```python
from build123d import *

# Parameters (mm, degrees)
SKETCH_1_R          = 1.600000000000001
SKETCH_1_R_2        = 1.6000000000000019
SKETCH_1_R_3        = 1.5999999999999985
EXTRUDE_1_DEPTH     = 3
EXTRUDE_2_DEPTH     = 30
CUT_EXTRUDE_1_DEPTH = 40
SKETCH_4_R          = 1.6499999999999986
SKETCH_4_R_2        = 1.6499999999999997
EXTRUDE_3_DEPTH     = 4
CUT_EXTRUDE_START   = -3
CUT_EXTRUDE_5_DEPTH = 3
EXTRUDE_4_DEPTH     = 3
FILLET_2_R          = 3
EXTRUDE_5_DEPTH     = 4
SKETCH_10_R         = 2.9999999999999996
CUT_EXTRUDE_6_DEPTH = 4
SKETCH_11_R         = 1.6500000000000008
CUT_EXTRUDE_7_DEPTH = 62.45571715470519


with BuildPart() as part:
    # 草图1 → 凸台-拉伸1 (new body)
    with BuildSketch(Plane.XY):
        with BuildLine():
            Line((-8.023322075989554, -14.631711796201198), (27.976677924010442, -14.631711796201193))
            Line((27.976677924010442, -14.631711796201193), (27.976677924010446, -38.631711796201195))
            Line((27.976677924010446, -38.631711796201195), (-8.023322075989551, -38.6317117962012))
            ThreePointArc((-8.023322075989551, -38.6317117962012), (-43.46930578748299, -14.57230150362017), (-57.14129859782335, 26.027570386525145))
            Line((-57.14129859782335, 26.027570386525145), (-34.48878313976992, 26.027570386525145))
            ThreePointArc((-34.48878313976992, 26.027570386525145), (-27.28963076602897, 1.7706236653637966), (-8.023322075989554, -14.631711796201198))
        make_face()
        with Locations((3.976677924010446, -26.6317117962012)):
            Circle(SKETCH_1_R, mode=Mode.SUBTRACT)
        with Locations(Location((15.976677924010446, -26.6317117962012, 0), (0, 0, 180))):
            Circle(SKETCH_1_R_2, mode=Mode.SUBTRACT)
        with Locations((-42.682604258715905, 20.02757038652514)):
            Circle(SKETCH_1_R_3, mode=Mode.SUBTRACT)
    extrude(amount=EXTRUDE_1_DEPTH)

    # 草图2 → 凸台-拉伸2 (add)
    with BuildSketch(Plane.XY.offset(3)):
        with BuildLine():
            Line((-20.49424577864387, -33.77498458475056), (-10.210218965484446, -13.591445522347069))
            ThreePointArc((-10.210218965484446, -13.591445522347069), (-5.231405442065514, -15.756295254952452), (-0.02587442417285965, -17.298243790895924))
            Line((-0.02587442417285965, -17.298243790895924), (-5.121581660002594, -39.370176745308015))
            ThreePointArc((-5.121581660002594, -39.370176745308015), (-12.979022025715798, -37.042696873124), (-20.49424577864387, -33.77498458475056))
        make_face()
    extrude(amount=EXTRUDE_2_DEPTH)

    # 草图3 → 切除-拉伸1 (cut)
    with BuildSketch(Plane.XY.offset(3)):
        with BuildLine():
            Line((-14.348702760927614, -28.820181203971632), (-7.456511566861831, -13.279984919997544))
            ThreePointArc((-7.456511566861831, -13.279984919997544), (-4.701142282615541, -14.38977235123981), (-1.875728376120071, -15.30668253882269))
            Line((-1.875728376120071, -15.30668253882269), (-6.561563425008877, -31.648131369774166))
            ThreePointArc((-6.561563425008877, -31.648131369774166), (-10.504001434072327, -30.368721805705025), (-14.348702760927614, -28.820181203971632))
        make_face()
    extrude(amount=CUT_EXTRUDE_1_DEPTH, mode=Mode.SUBTRACT)

    # 草图4 → 凸台-拉伸3 (add)
    with BuildSketch(Plane.XY.offset(33)):
        Polygon((-27.87837659400939, -26.811760111104594), (5.010865133497435, -38.782465127502874), (27.24217444966564, 22.297555223581274), (16.435709310627683, 26.230786871826414), (-0.6652978556555434, -20.753844167469087), (-11.941609305086462, -16.649602447561108), (-15.43021476700824, -26.234467179577372), (-26.236679906046202, -22.30123553133223), align=None)
        with Locations((20.36376431871485, 19.48020290794287)):
            Circle(SKETCH_4_R, mode=Mode.SUBTRACT)
        with Locations((0.4581919771611356, -35.20990762179707)):
            Circle(SKETCH_4_R_2, mode=Mode.SUBTRACT)
        with Locations(Location((-22.094430921700695, -27.001424181981108, 0), (0, 0, 180))):
            Circle(SKETCH_4_R, mode=Mode.SUBTRACT)
    extrude(amount=EXTRUDE_3_DEPTH)

    # 草图7 → 切除-拉伸5 (cut)
    with BuildSketch(Plane.XY.offset(3).offset(CUT_EXTRUDE_START)):
        with BuildLine():
            Line((-12.256052607879635, -12.480648485696536), (-23.582310336906296, -32.09830233199053))
            ThreePointArc((-23.582310336906296, -32.09830233199053), (-48.149194794505114, -7.53141787439181), (-57.14129859782335, 26.027570386525152))
            Line((-57.14129859782335, 26.027570386525152), (-34.48878313976992, 26.027570386525145))
            ThreePointArc((-34.48878313976992, 26.027570386525145), (-28.53154094821116, 3.794839854634926), (-12.256052607879635, -12.480648485696536))
        make_face()
    extrude(amount=CUT_EXTRUDE_5_DEPTH, mode=Mode.SUBTRACT)

    # 草图8 → 凸台-拉伸4 (add)
    with BuildSketch(Plane(origin=(0, 0, 0), x_dir=(-1, 0, 0), z_dir=(0, 0, -1))):
        with BuildLine():
            Line((-27.976677924010446, -38.631711796201195), (8.023322075989551, -38.6317117962012))
            ThreePointArc((8.023322075989551, -38.6317117962012), (-9.97667792401045, -41.090406135308655), (-27.976677924010446, -38.631711796201195))
        make_face()
    extrude(amount=-EXTRUDE_4_DEPTH)

    # 圆角2
    fillet_2_edges = [part.edges().sort_by_distance(p)[0] for p in [
        (-26.236679906046202, -22.30123553133223, 35),
    ]]
    fillet(fillet_2_edges, radius=FILLET_2_R)
    fillet_2_2_edges = [part.edges().sort_by_distance(p)[0] for p in [
        (27.24217444966564, 22.297555223581274, 35),
    ]]
    fillet(fillet_2_2_edges, radius=FILLET_2_R)
    fillet_2_3_edges = [part.edges().sort_by_distance(p)[0] for p in [
        (16.435709310627683, 26.230786871826414, 35),
    ]]
    fillet(fillet_2_3_edges, radius=FILLET_2_R)
    fillet_2_4_edges = [part.edges().sort_by_distance(p)[0] for p in [
        (27.976677924010446, -38.631711796201195, 1.5),
    ]]
    fillet(fillet_2_4_edges, radius=FILLET_2_R)
    fillet_2_5_edges = [part.edges().sort_by_distance(p)[0] for p in [
        (-23.5823103369063, -32.09830233199054, 1.5),
    ]]
    fillet(fillet_2_5_edges, radius=FILLET_2_R)
    fillet_2_6_edges = [part.edges().sort_by_distance(p)[0] for p in [
        (-12.256052607879633, -12.480648485696538, 1.5),
    ]]
    fillet(fillet_2_6_edges, radius=FILLET_2_R)
    fillet_2_7_edges = [part.edges().sort_by_distance(p)[0] for p in [
        (27.976677924010442, -14.631711796201193, 1.5),
    ]]
    fillet(fillet_2_7_edges, radius=FILLET_2_R)
    # the kernel refuses this fillet: 3 mm, written as the material it adds along each edge
    with BuildSketch(Plane(origin=(-0.6652978556555434, -20.753844167469087, 33), x_dir=(-0.93969262078591, 0.34202014332566444, 0), z_dir=(0, 0, 1))) as fillet_2_8_piece_1:
        with BuildLine():
            CenterArc((FILLET_2_R, -FILLET_2_R), FILLET_2_R, 89.99999999999999, 90.00000000000001)
            Line((5e-17, -FILLET_2_R), (-FILLET_2_R * 0.02, -FILLET_2_R))
            Line((-FILLET_2_R * 0.02, -FILLET_2_R), (-FILLET_2_R * 0.02, FILLET_2_R * 0.02))
            Line((-FILLET_2_R * 0.02, FILLET_2_R * 0.02), (FILLET_2_R, FILLET_2_R * 0.02))
            Line((FILLET_2_R, FILLET_2_R * 0.02), (FILLET_2_R, -5e-17))
        make_face()
    extrude(amount=4)
    # the kernel refuses this fillet: 3 mm, written as the material it takes off along each edge
    with BuildSketch(Plane(origin=(-11.941609305086462, -16.649602447561108, 33), x_dir=(0.9396926207859099, -0.3420201433256647, 0), z_dir=(0, 0, 1))) as fillet_2_9_piece_1:
        with BuildLine():
            CenterArc((FILLET_2_R, -FILLET_2_R), FILLET_2_R, 89.99999999999997, 90)
            Line((-2.84e-15, -FILLET_2_R), (-FILLET_2_R * 0.02, -FILLET_2_R))
            Line((-FILLET_2_R * 0.02, -FILLET_2_R), (-FILLET_2_R * 0.02, FILLET_2_R * 0.02))
            Line((-FILLET_2_R * 0.02, FILLET_2_R * 0.02), (FILLET_2_R, FILLET_2_R * 0.02))
            Line((FILLET_2_R, FILLET_2_R * 0.02), (FILLET_2_R, -5e-17))
        make_face()
    extrude(amount=11.5, mode=Mode.SUBTRACT)
    # the kernel refuses this fillet: 3 mm, written as the material it adds along each edge
    with BuildSketch(Plane(origin=(-15.43021476700824, -26.234467179577372, 33), x_dir=(0.34202014332566544, 0.9396926207859095, 0), z_dir=(0, 0, 1))) as fillet_2_10_piece_1:
        with BuildLine():
            CenterArc((FILLET_2_R, FILLET_2_R), FILLET_2_R, 180.00000000000006, 90)
            Line((-5.63e-15, FILLET_2_R), (-FILLET_2_R * 0.02, FILLET_2_R))
            Line((-FILLET_2_R * 0.02, FILLET_2_R), (-FILLET_2_R * 0.02, -FILLET_2_R * 0.02))
            Line((-FILLET_2_R * 0.02, -FILLET_2_R * 0.02), (FILLET_2_R, -FILLET_2_R * 0.02))
            Line((FILLET_2_R, -FILLET_2_R * 0.02), (FILLET_2_R, 9e-17))
        make_face()
    extrude(amount=4)

    # 草图9 → 凸台-拉伸5 (add)
    with BuildSketch(Plane.XY.offset(37.00000000000001)):
        with BuildLine():
            Line((-27.87837659400939, -26.811760111104594), (-29.094175630850113, -30.152140511419198))
            ThreePointArc((-29.094175630850113, -30.152140511419198), (-13.427826993623084, -38.27577838818826), (3.79506609665671, -42.12284552781748))
            Line((3.79506609665671, -42.12284552781748), (5.010865133497435, -38.782465127502874))
            Line((5.010865133497435, -38.782465127502874), (-27.87837659400939, -26.811760111104594))
        make_face()
    extrude(amount=-EXTRUDE_5_DEPTH)

    # 草图10 → 切除-拉伸6 (cut)
    with BuildSketch(Plane.XY.offset(37.00000000000001)):
        with Locations((3.976677924010446, -26.6317117962012)):
            Circle(SKETCH_10_R)
    extrude(amount=-CUT_EXTRUDE_6_DEPTH, mode=Mode.SUBTRACT)

    # 草图11 → 切除-拉伸7 (cut, through all)
    with BuildSketch(Plane.XY.offset(3)):
        with Locations((0.4581919771611356, -35.20990762179707)):
            Circle(SKETCH_11_R)
    extrude(amount=-CUT_EXTRUDE_7_DEPTH, mode=Mode.SUBTRACT)


solid = part.part
```
Read the model definition and answer for the solid it produces. Units are mm, in the model's axes. A direction names the side the tool comes from. Coordinates: 2 decimals unless noted, no trailing zeros. Loops run counter-clockwise (first coordinate to the right, second up) from the corner with the lowest first, then second, coordinate; pieces in that order, holes last.
(1) The part is cut by section D-D (y = 15). Determine the outline of the cut face in (x, z).
Solution:
outline: (12.35, 33) - (24.59, 33) - (24.59, 37) - (12.35, 37) - close
(2) Flat-ended cylindrical pins translate along their axes: pin 1 Ø6 at (x, y) = (18, -33) entering from +Z; pin 2 Ø8 at (y, z) = (8, 30) entering from -X; pin 3 Ø3 at (y, z) = (-17, 11) entering from -X. Find the tip coordinate at first contact, or state that the pin passes through.
Solution:
pin 1: stops at z = 3
pin 2: stops at x = 8.84
pin 3: stops at x = -12.71
(3) The mould has two halves that part along Y. Classify faces 5 (the face through (-2, -18, 33)), 6 (the face through (-10.45, -30.39, 17.79)), 7 (the face through (27.075, -15.487, 1.521)), 8 (the face through (1.22, -36.674, 34.972)): released by +Y, released by -Y, zero draft, split by the parting line, or undercut.
Solution:
face 5: zero draft
face 6: undercut
face 7: released by +Y
face 8: undercut
(4) The part is cut by section A-A (z = 16.5). Determine the outline of the cut face in (x, y).
Solution:
outline: (-20.49, -33.77) arc R67.12 ccw to (-5.12, -39.37) - (-0.03, -17.3) arc R44.47 cw to (-2.28, -16.72) - (-6.56, -31.65) arc R60 cw to (-14.35, -28.82) - (-8.05, -14.62) arc R44.47 cw to (-9.78, -13.81) arc R3 ccw to (-10.23, -13.63) - close
(5) The part is cut by section C-C (y = -21.5). Determine the outline of the cut face in (x, z).
Solution:
outline: (-17.46, 0) - (27.98, 0) - (27.98, 3) - (-1, 3) - (-1, 33) - (11.3, 33) - (11.3, 37) - (-13.71, 37) - (-13.71, 33) - (-14.24, 33) - (-14.24, 3) - (-17.46, 3) - close; hole (-11.1, 3) - (-3.65, 3) - (-3.65, 33) - (-11.1, 33) - close
(6) Consider line 1 along Z through (x, y) = (-12, -28); line 2 along X through (y, z) = (-21.5, 5.5); line 3 along Z through (x, y) = (10.5, -38). Determine where each line is inside the solid, lowest interval first.
Solution:
line 1: z = 0 to 3, 33 to 37
line 2: x = -14.24 to -11.1, -3.65 to -1
line 3: z = 0 to 3
(7) A tool of negligible diameter and unlimited length cuts with its end or side. For faces 1 (the face through (-15.43, -23.84, 17.79)), 2 (the face through (-15.985, -25.122, 34.972)), 3 (the face through (-11.244, -21.819, 17.79)), 4 (the face through (3.33, -29.56, 35.03)), from which of +Z, -Z, +X, -X, +Y, -Y can it reach the whole face along a straight path? Write none if from no direction.
Solution:
face 1: -X, +Y
face 2: +Z, +Y
face 3: none
face 4: +Z
(8) The part is cut by section B-B (x = -11). Determine the outline of the cut face in (y, z), and give its area (3 significant figures).
Solution:
outline: (-39.11, 33) - (-37.73, 33) - (-37.73, 0) - (-13.5, 0) - (-13.5, 3) - (-15.14, 3) - (-15.14, 33) - (-17.62, 33) - (-17.62, 37) - (-39.11, 37) - close; hole (-30.19, 3) - (-21.27, 3) - (-21.27, 33) - (-30.19, 33) - close
area: 569 mm2
